Model file for the job. Use its own axes, mm. Coordinates: 2 decimals unless noted, no trailing zeros. Write each loop counter-clockwise with the first axis right and the second up, starting at its lowest first coordinate (ties: lowest second). Pieces come first, ordered by that corner, then holes.
Q1. Band-saw the part on A-A, the plane x = 191.5. Write the cut outline in (y, z).
Q2. Pull direction Y, two halves, no side cores. Call faces 1 (the cylindrical face through (84.646, 14.042, 1.479)), 2 (the flat face through (175, 16, 3)), 3 (the cylindrical face through (122.8, 14.72, 1.48)): released by +Y, released by -Y, zero draft, split by the parting line, or undercut.
Q3. Pin check, flat tips, straight feed: P1, Ø5.5, axis at x = 26.63, y = 15.87, coming from the -Z side; P2, Ø1.5, axis at y = 16, z = 2, coming from the +X side; P3, Ø8, axis at x = 37.63, y = 15.87, coming from the -Z side. Stop position of each tip, or through.
Q4. Drill centre lines: probe 1 along Y at (x, z) = (191, 2.7); probe 2 along Y at (x, z) = (204, 1.85). Where is each one in solid material? Low to high.
Q5. Band-saw the part on B-B, the plane z = 1.25. State how many separate pieces and enclosed holes the cut face has, plus the area to 3 significant figures.
from build123d import *

# Parameters (mm, degrees)
MODEL_R         = 3
MODEL_W         = 1.5
MODEL_H         = 5
MODEL_W_2       = 2
MODEL_H_2       = 3
EXTRUDE_1_DEPTH = 3


with BuildPart() as part:
    # Model → 凸台-拉伸1 (new body)
    with BuildSketch(Plane.XY):
        Polygon((13.851287916, 22.788853141), (13.851287916, 18.367254581), (15.851287916, 18.367254581), (15.851287916, 13.367254581), (13.851287916, 13.367254581), (13.851287916, 8.945653722), (29.822931445, 8.945653722), (340.851287916, 8.945653722), (340.851287916, 13.367254581), (338.851287916, 13.367254581), (338.851287916, 18.367254581), (340.851287916, 18.367254581), (340.851287916, 22.788853141), (29.824992994, 22.788853141), align=None)
        with Locations((26.631213357, 15.867254581)):
            Circle(MODEL_R, mode=Mode.SUBTRACT)
        with Locations((37.631213357, 15.867254581)):
            Circle(MODEL_R, mode=Mode.SUBTRACT)
        with Locations((48.631213357, 15.867254581)):
            Circle(MODEL_R, mode=Mode.SUBTRACT)
        with Locations((59.631213357, 15.867254581)):
            Circle(MODEL_R, mode=Mode.SUBTRACT)
        with Locations((70.631213357, 15.867254581)):
            Circle(MODEL_R, mode=Mode.SUBTRACT)
        with Locations((87.026286184, 15.867254581)):
            Circle(MODEL_R, mode=Mode.SUBTRACT)
        with Locations((98.026286184, 15.867254581)):
            Circle(MODEL_R, mode=Mode.SUBTRACT)
        with Locations((109.026286184, 15.867254581)):
            Circle(MODEL_R, mode=Mode.SUBTRACT)
        with Locations((120.026286184, 15.867254581)):
            Circle(MODEL_R, mode=Mode.SUBTRACT)
        with Locations((133.205424602, 15.867254581)):
            Circle(MODEL_R, mode=Mode.SUBTRACT)
        with Locations((144.205424602, 15.867254581)):
            Circle(MODEL_R, mode=Mode.SUBTRACT)
        with Locations((155.205424602, 15.867254581)):
            Circle(MODEL_R, mode=Mode.SUBTRACT)
        with Locations((166.205424602, 15.867254581)):
            Circle(MODEL_R, mode=Mode.SUBTRACT)
        with Locations((180.575631043, 15.867254581)):
            Circle(MODEL_R, mode=Mode.SUBTRACT)
        with Locations((191.575631043, 15.867254581)):
            Circle(MODEL_R, mode=Mode.SUBTRACT)
        with Locations((202.575631043, 15.867254581)):
            Circle(MODEL_R, mode=Mode.SUBTRACT)
        with Locations((220.335604036, 15.867254581)):
            Circle(MODEL_R, mode=Mode.SUBTRACT)
        with Locations((231.335604036, 15.867254581)):
            Circle(MODEL_R, mode=Mode.SUBTRACT)
        with Locations((242.335604036, 15.867254581)):
            Circle(MODEL_R, mode=Mode.SUBTRACT)
        with Locations((253.335604036, 15.867254581)):
            Circle(MODEL_R, mode=Mode.SUBTRACT)
        with Locations((264.335604036, 15.867254581)):
            Circle(MODEL_R, mode=Mode.SUBTRACT)
        with Locations((285.040254887, 15.867254581)):
            Circle(MODEL_R, mode=Mode.SUBTRACT)
        with Locations((296.040254887, 15.867254581)):
            Circle(MODEL_R, mode=Mode.SUBTRACT)
        with Locations((307.040254887, 15.867254581)):
            Circle(MODEL_R, mode=Mode.SUBTRACT)
        with Locations((318.040254887, 15.867254581)):
            Circle(MODEL_R, mode=Mode.SUBTRACT)
        with Locations((329.040254887, 15.867254581)):
            Circle(MODEL_R, mode=Mode.SUBTRACT)
        with Locations((79.851287916, 15.867254581)):
            Rectangle(MODEL_W, MODEL_H, mode=Mode.SUBTRACT)
        with Locations((209.851287916, 15.867254581)):
            Rectangle(MODEL_W, MODEL_H, mode=Mode.SUBTRACT)
        with Locations((274.851287916, 15.867254581)):
            Rectangle(MODEL_W, MODEL_H, mode=Mode.SUBTRACT)
        with Locations((172.851287916, 15.87827705)):
            Rectangle(MODEL_W_2, MODEL_H_2, mode=Mode.SUBTRACT)
        with Locations((127.351287916, 15.867254581)):
            Rectangle(MODEL_W, MODEL_H, mode=Mode.SUBTRACT)
    extrude(amount=EXTRUDE_1_DEPTH)


solid = part.part
Answer sheet:
1. outline: (8.95, 0) - (12.87, 0) - (12.87, 3) - (8.95, 3) - close; (18.87, 0) - (22.79, 0) - (22.79, 3) - (18.87, 3) - close
2. face 1: undercut
2. face 2: zero draft
2. face 3: undercut
3. P1: passes through
3. P2: stops at x = 338.85
3. P3: stops at z = 0
4. probe 1: y = 8.95 to 12.92, 18.81 to 22.79
4. probe 2: y = 8.95 to 13.23, 18.51 to 22.79
5. separate pieces: 1
5. enclosed holes: 31
5. area: 3,740 mm2
